For this review, use the dimensioned drawing (mm, ordinates from the lowest corner) and the shaded views. Round coordinates to 2 decimals unless told otherwise and drop trailing zeros. Write each loop counter-clockwise with the first axis right and the second up, starting at its lowest first coordinate (ties: lowest second). Pieces come first, ordered by that corner, then holes. Notation, with made-up numbers: (-29.75, 71) - (10.25, 71) arc R9 ccw to (10.25, 88) - close; hole circle Ø7 at (39.5, -7.75). An arc over 180 degrees is marked (long way). Return JSON: item names as keys, results as strings.
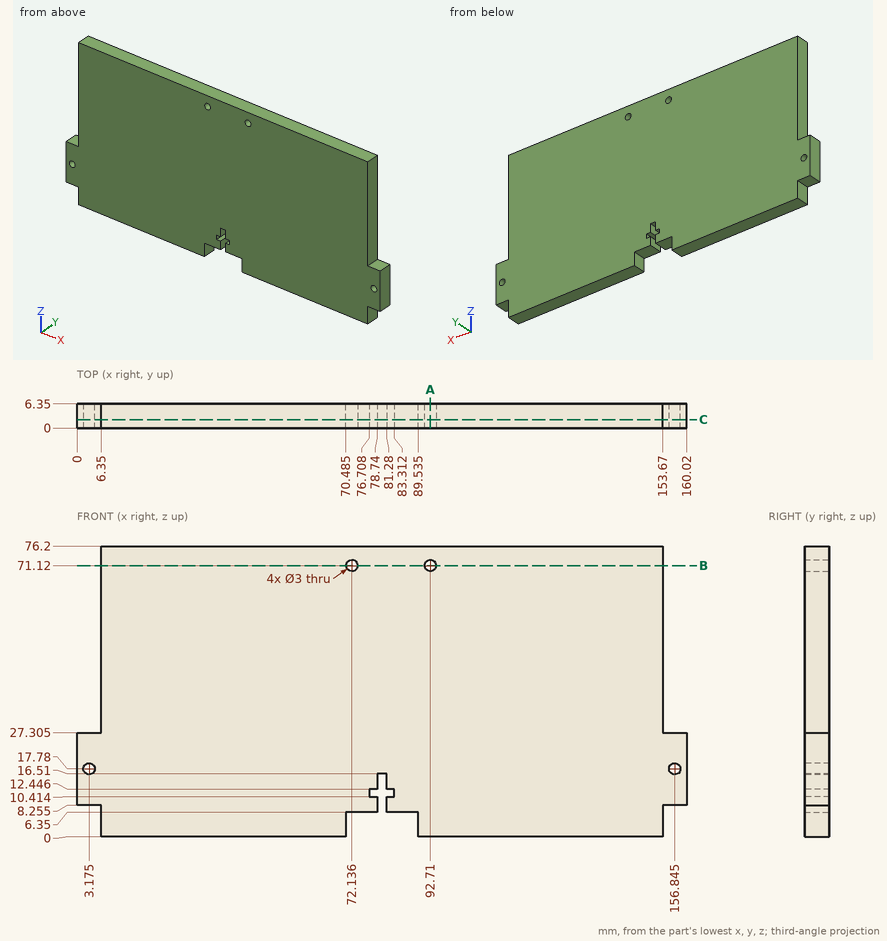
(1) Add section A-A (x = 92.71). Write out the cut boundary in (y, z).
Filled in:
{"outline": "(0, 0) - (6.35, 0) - (6.35, 69.62) - (0, 69.62) - close; (0, 72.62) - (6.35, 72.62) - (6.35, 76.2) - (0, 76.2) - close"}
(2) Wall thickness on line 1 (X direction, y = 3, z = 71.12); line 2 (X direction, y = 2.75, z = 6) (3 decimals); line 3 (X direction, y = 2.75, z = 16): over which ranges is each line inside the solid? List them lowest first.
Filled in:
{"line 1": "x = 6.35 to 70.64, 73.64 to 91.21, 94.21 to 153.67", "line 2": "x = 6.35 to 70.485, 89.535 to 153.67", "line 3": "x = 0 to 78.74, 81.28 to 160.02"}
(3) Add section B-B (z = 71.12). Write out the cut boundary in (x, y), plus the area to 3 significant figures.
Filled in:
{"outline": "(6.35, 0) - (70.64, 0) - (70.64, 6.35) - (6.35, 6.35) - close; (73.64, 0) - (91.21, 0) - (91.21, 6.35) - (73.64, 6.35) - close; (94.21, 0) - (153.67, 0) - (153.67, 6.35) - (94.21, 6.35) - close", "area": "897 mm2"}
(4) Add section C-C (y = 2.25). Give the number of separate pieces and of enclosed holes in the cut face, plus the area to 3 significant figures.
Filled in:
{"separate pieces": "1", "enclosed holes": "4", "area": "11,300 mm2"}
(5) Clearance check with flat-ended pins moving along their axes: pin 1 Ø1 at (y, z) = (5, 65.5) entering from +X; pin 2 Ø2.5 at (x, z) = (72.136, 71.12) entering from -Y; pin 3 Ø3 at (y, z) = (1.5, 4.5) entering from -X; pin 4 Ø3 at (x, y) = (3, 4) entering from +Z (3 decimals). State where each tip first meets the part, or that it passes through.
Filled in:
{"pin 1": "stops at x = 153.67", "pin 2": "passes through", "pin 3": "stops at x = 6.35", "pin 4": "stops at z = 27.305"}
